```python
from build123d import *

# Parameters (mm, degrees)
SKETCH1_R           = 1.5
SKETCH1_R_2         = 2
BOSS_EXTRUDE1_DEPTH = 5


with BuildPart() as part:
    # Sketch1 → Boss-Extrude1 (new body)
    with BuildSketch(Plane.XY):
        with BuildLine():
            ThreePointArc((35.408332353, -6.5), (0, 36), (-35.408332353, -6.5))
            Line((-35.408332353, -6.5), (-7.998604295, -6.5))
            Line((-7.998604295, -6.5), (-7.998604295, 0))
            ThreePointArc((-7.998604295, 0), (0, 7.998604295), (7.998604295, 0))
            Line((7.998604295, 0), (7.998604295, -6.5))
            Line((7.998604295, -6.5), (35.408332353, -6.5))
        make_face()
        with Locations((-32.5, 0)):
            Circle(SKETCH1_R, mode=Mode.SUBTRACT)
        with Locations((-11.313708499, 0)):
            Circle(SKETCH1_R_2, mode=Mode.SUBTRACT)
        with Locations((0, 11.313708499)):
            Circle(SKETCH1_R_2, mode=Mode.SUBTRACT)
        with Locations((11.313708499, 0)):
            Circle(SKETCH1_R_2, mode=Mode.SUBTRACT)
        with Locations((32.5, 0)):
            Circle(SKETCH1_R, mode=Mode.SUBTRACT)
        with Locations((-16.25, 28.145825623)):
            Circle(SKETCH1_R, mode=Mode.SUBTRACT)
        with Locations((16.25, 28.145825623)):
            Circle(SKETCH1_R, mode=Mode.SUBTRACT)
    extrude(amount=BOSS_EXTRUDE1_DEPTH)


solid = part.part
```
Build history of the part. All positions in model axes, mm. A direction names the side the tool comes from. Round coordinates to 2 decimals unless told otherwise and drop trailing zeros. Write each loop counter-clockwise with the first axis right and the second up, starting at its lowest first coordinate (ties: lowest second). Pieces come first, ordered by that corner, then holes. Notation, with made-up numbers: (-28.75, 58.25) - (3.25, 58.25) arc R16 cw to (3.25, 68.25) - close; hole circle Ø2 at (-13, 34.25). An arc over 180 degrees is marked (long way). Answer as CSV lines item,"result".
Q1. Tool access for faces 1 (the flat face through (7.999, -3, 2)), 2 (the flat face through (-1, 15, 0)): list every direction of +Z, -Z, +X, -X, +Y, -Y with a clear straight run to the whole face (end or side of a thin tool).
Report:
face 1,"+Z, -Z, -Y"
face 2,"-Z, +X, -X, +Y, -Y"
Q2. Cut at A-A (x = 16.25). Write the cut outline in (y, z), and give its area (3 significant figures).
Report:
outline,"(-6.5, 0) - (26.65, 0) - (26.65, 5) - (-6.5, 5) - close; (29.65, 0) - (32.12, 0) - (32.12, 5) - (29.65, 5) - close"
area,"178 mm^2"
Q3. Cut at D-D (y = 17). Write the cut outline in (x, z), and give its area (3 significant figures).
Report:
outline,"(-31.73, 0) - (31.73, 0) - (31.73, 5) - (-31.73, 5) - close"
area,"317 mm^2"
Q4. Cut at C-C (x = 32.5). Write the cut outline in (y, z).
Report:
outline,"(-6.5, 0) - (-1.5, 0) - (-1.5, 5) - (-6.5, 5) - close; (1.5, 0) - (15.48, 0) - (15.48, 5) - (1.5, 5) - close"
Q5. Cut at B-B (z = 1.6). Write the cut outline in (x, y), and give its area (3 significant figures).
Report:
outline,"(-35.41, -6.5) - (-8, -6.5) - (-8, 0) arc R8 cw to (8, 0) - (8, -6.5) - (35.41, -6.5) arc R36 ccw (long way) to start; hole circle Ø3 at (-32.5, 0); hole circle Ø3 at (-16.25, 28.15); hole circle Ø4 at (-11.31, 0); hole circle Ø4 at (0, 11.31); hole circle Ø4 at (11.31, 0); hole circle Ø3 at (16.25, 28.15); hole circle Ø3 at (32.5, 0)"
area,"2,230 mm^2"
Q6. Pull direction Y, two halves, no side cores. Call faces 3 (the flat face through (-7.999, -3, 2)), 4 (the cylindrical face through (-16.575, 26.681, 2.465)), 5 (the cylindrical face through (0, 8, 2)): +Y half, -Y half, draft (parallel to the pull), parting line (faces both ways), or undercut.
Report:
face 3,"draft"
face 4,"undercut"
face 5,"-Y half"
Q7. Drop flat-ended pins along their axis: pin 1 (1 mm diameter, centred on y = 17.5, z = 3.5, fed in from -X); pin 2 (1.5 mm diameter, centred on y = -4, z = 2.5, fed in from +X); pin 3 (1.5 mm diameter, centred on y = 31.5, z = 2, fed in from +X). Give the stop position or say it passes through.
Report:
pin 1,"stops at x = -31.73"
pin 2,"stops at x = 35.85"
pin 3,"stops at x = 18.72"
Q8. Drill centre lines: probe 1 along X at (y, z) = (27, 4.55); probe 2 along X at (y, z) = (6.5, 4.8); probe 3 along X at (y, z) = (29.5, 4.7). Where is each one in solid material? Low to high. Write a range as [from, to].
Report:
probe 1,"x = [-23.81, -17.22], [-15.28, 15.28], [17.22, 23.81]"
probe 2,"x = [-35.41, -4.66], [4.66, 35.41]"
probe 3,"x = [-20.63, -16.9], [-15.6, 15.6], [16.9, 20.63]"
